Read the model definition and answer for the solid it produces. Units are mm, in the model's axes. A direction names the side the tool comes from. Give positions to 0.01 mm unless a question says otherwise; leave off trailing zeros. Loops run counter-clockwise (first coordinate to the right, second up) from the corner with the lowest first, then second, coordinate; pieces in that order, holes last. Notation, with made-up numbers: (-3.5, 1) - (2.5, 1) arc R13 ccw to (2.5, 23) - close; hole circle Ø9 at (35.5, 83.5). An arc over 180 degrees is marked (long way). Put each result on its own line as item: value. Start each with the question number.
1. A cutting plane is placed at A-A, the plane x = 18. Determine the outline of the cut face in (y, z).
2. A cutting plane is placed at B-B, the plane z = 0. Determine the outline of the cut face in (x, y), plus the area to 3 significant figures.
3. For faces 1 (the flat face through (17.452, -21.483, 21.734)), 2 (the flat face through (13.589, 0, 0)), determine the directions among +Z, -Z, +X, -X, +Y, -Y from which every point of the face is accessible in a straight line to the end or side of a thin tool.
4. Consider L1, parallel to Z at x = -8, y = 0; L2, parallel to X at y = 13.5, z = 21. Determine where each line is inside the solid, lowest interval first. Write a range as from..to.
5. A cutting plane is placed at C-C, the plane x = -15. Determine the outline of the cut face in (y, z) (1 decimal).
6. Given pin 1 Ø6 at (x, y) = (13.5, 22) entering from -Z; pin 2 Ø6 at (x, y) = (3.5, 6) entering from -Z; pin 3 Ø8 at (x, z) = (14, 13.5) entering from +Y; pin 4 Ø12 at (x, z) = (-7.5, -22) entering from -Y, each flat-ended and moving along its own axis, determine where each tip first touches the part or whether it passes through.
7. For a pull along Z with two mould halves and no side action, classify faces 3 (the cylindrical face through (-4.054, 3.417, -26.028)), 4 (the flat face through (17, 0, 30.559)), 5 (the flat face through (-21.209, -9, -25)) as released by +Z, released by -Z, zero draft, split by the parting line, or undercut.
```python
from build123d import *

# Parameters (mm, degrees)
SKETCH2_R           = 30.1625
BOSS_EXTRUDE1_DEPTH = 7.62


with BuildPart() as part:
    # Sketch1 → Revolve1 (revolve)
    with BuildSketch(Plane.XY):
        Polygon((-21.209, -30.1625), (21.209, -30.1625), (21.209, 0), (13.589, 0), (13.589, -26.2509), (-21.209, -26.2509), align=None)
    revolve(axis=Axis((-21.209, 0, 0), (1, 0, 0)))

    # Sketch2 → Boss-Extrude1 (add)
    with BuildSketch(Plane(origin=(21.209, 0, 0), x_dir=(0, 0, -1), z_dir=(1, 0, 0))):
        Polygon((-12.658107583, 30.559375), (-30.559375, 12.658107583), (-30.559375, -12.658107583), (-12.658107583, -30.559375), (12.658107583, -30.559375), (30.559375, -12.658107583), (30.559375, 12.658107583), (12.658107583, 30.559375), align=None)
        Circle(SKETCH2_R, mode=Mode.SUBTRACT)
    extrude(amount=-BOSS_EXTRUDE1_DEPTH)


solid = part.part
```
Return value:
1. outline: (-30.56, -12.66) - (-12.66, -30.56) - (12.66, -30.56) - (30.56, -12.66) - (30.56, 12.66) - (12.66, 30.56) - (-12.66, 30.56) - (-30.56, 12.66) - close
2. outline: (-21.21, -30.16) - (13.59, -30.16) - (13.59, -30.56) - (21.21, -30.56) - (21.21, 30.56) - (13.59, 30.56) - (13.59, 30.16) - (-21.21, 30.16) - (-21.21, 26.25) - (13.59, 26.25) - (13.59, -26.25) - (-21.21, -26.25) - close
2. area: 738 mm2
3. face 1: +Z, +X, -X, -Y
3. face 2: -X
4. L1: z = -30.16..-26.25, 26.25..30.16
4. L2: x = 13.59..21.21
5. outline: circle Ø60.3 at (0, 0); hole circle Ø52.5 at (0, 0)
6. pin 1: stops at z = -24.22
6. pin 2: stops at z = -30.01
6. pin 3: stops at y = 30.56
6. pin 4: stops at y = -25.57
7. face 3: undercut
7. face 4: released by +Z
7. face 5: zero draft
